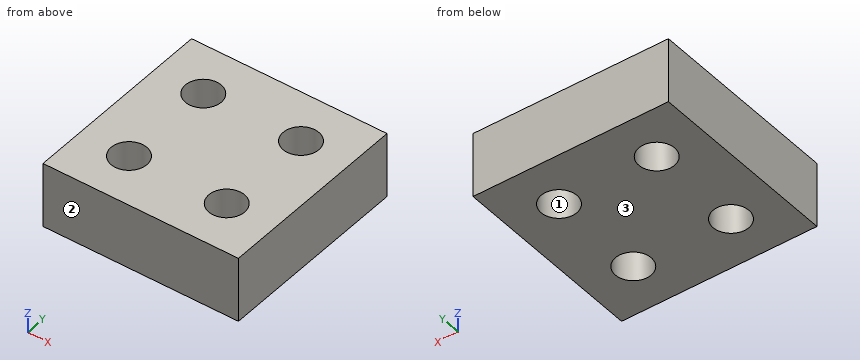
Solid Edge part; units mm, degrees
sketch "Sketch1" plane through (0, 0, 0) normal (0, 0, 1) x (1, 0, 0)
  circle A0 centre (6, 6) radius 2.2
  circle A1 centre (6, -6) radius 2.2
  circle A2 centre (-6, -6) radius 2.2
  line L0 (-12, -12) -> (12, -12)
  line L1 (12, -12) -> (12, 12)
  line L2 (12, 12) -> (-12, 12)
  line L3 (-12, 12) -> (-12, -12)
  circle A3 centre (-6, 6) radius 2.2
  dimension "D1" = 12
  dimension "D2" = 12
extrude "Protrusion1" add sketch "Sketch1" along normal blind 8
properties material "ABS Plastic, medium impact"
Verification items for the finished model (mm, model axes). Face numbers are marked on the shaded views. Give positions to 0.01 mm unless a question says otherwise; leave off trailing zeros. Loops run counter-clockwise (first coordinate to the right, second up) from the corner with the lowest first, then second, coordinate; pieces in that order, holes last.
1. Thickness scan on line 1 (Y direction, x = -6, z = 4.5); line 2 (X direction, y = -5, z = 7); line 3 (Y direction, x = 6.5, z = 4). Record the ranges inside material, lowest first.
2. Section check B-B, the plane z = 3.5. Enter the section's corners in (x, y), then the cut area to 3 significant figures.
3. Section check C-C, the plane x = 4.75. Enter the section's corners in (y, z), then the cut area to 3 significant figures.
4. Mould release check, pull along Y, two halves, no side actions. Record for the marked faces 1, 2 and 3: released by +Y, released by -Y, zero draft, split by the parting line, or undercut.
5. Section check A-A, the plane x = -6. Enter the section's corners in (y, z), then the cut area to 3 significant figures.
6. Go/stop test with a flat-tipped pin: pin 1 Ø3.5 at (x, y) = (-6, -6) entering from +Z. Record where the tip stops, or that it passes through.
Geometry says:
1. line 1: y = -12 to -8.2, -3.8 to 3.8, 8.2 to 12
1. line 2: x = -12 to -7.96, -4.04 to 4.04, 7.96 to 12
1. line 3: y = -12 to -8.14, -3.86 to 3.86, 8.14 to 12
2. outline: (-12, -12) - (12, -12) - (12, 12) - (-12, 12) - close; hole circle Ø4.4 at (-6, -6); hole circle Ø4.4 at (-6, 6); hole circle Ø4.4 at (6, -6); hole circle Ø4.4 at (6, 6)
2. area: 515 mm2
3. outline: (-12, 0) - (-7.81, 0) - (-7.81, 8) - (-12, 8) - close; (-4.19, 0) - (4.19, 0) - (4.19, 8) - (-4.19, 8) - close; (7.81, 0) - (12, 0) - (12, 8) - (7.81, 8) - close
3. area: 134 mm2
4. face 1: undercut
4. face 2: released by -Y
4. face 3: zero draft
5. outline: (-12, 0) - (-8.2, 0) - (-8.2, 8) - (-12, 8) - close; (-3.8, 0) - (3.8, 0) - (3.8, 8) - (-3.8, 8) - close; (8.2, 0) - (12, 0) - (12, 8) - (8.2, 8) - close
5. area: 122 mm2
6. pin 1: passes through
